Autodesk Inventor part; units mm, degrees
ref_plane "YZ Plane" through (0, 0, 0) normal (1, 0, 0) x (0, 1, 0)
ref_plane "XZ Plane" through (0, 0, 0) normal (0, 1, 0) x (-1, 0, 0)
ref_plane "XY Plane" through (0, 0, 0) normal (0, 0, 1) x (1, 0, 0)
sketch "スケッチ1" plane through (0, 0, 0) normal (0, 0, 1) x (1, 0, 0)
  circle A0 centre (0, 0) radius 1.5
  dimension "d0" = 3
extrude "押し出し1" add sketch "スケッチ1" along normal blind 6
sketch "スケッチ2" plane through (0, 0, 6) normal (0, 0, 1) x (1, 0, 0)
  circle A0 centre (0, 0) radius 1.5
  circle A1 centre (0, 0) radius 3
  dimension "d3" = 6
extrude "押し出し2" add sketch "スケッチ2" along normal blind 2 contours A0 | A1
fillet "フィレット1" radius 2 1 edges at (-3, 0, 8)
thread "ねじ1"
sketch "スケッチ3" plane through (0, 0, 0) normal (0, 0, -1) x (-1, 0, 0)
  circle A0 centre (0, 0) radius 1.5
extrude "押し出し3" add sketch "スケッチ3" along normal blind 9
sketch "スケッチ4" plane through (0, 0, -9) normal (0, 0, -1) x (-1, 0, 0)
  circle A0 centre (0, 0) radius 1.5
extrude "押し出し4" add sketch "スケッチ4" along normal blind 15
properties part number "SB　30mmなべネジ" material "Steel, Mild"
Design review of the part built by this model. Coordinates are the model's own, in mm. A direction names the side the tool comes from. Coordinates: 2 decimals unless noted, no trailing zeros. Loops run counter-clockwise (first coordinate to the right, second up) from the corner with the lowest first, then second, coordinate; pieces in that order, holes last.
Item 1: Add section A-A (z = -2.5). Write out the cut boundary in (x, y), and give its area (3 significant figures).
Completed:
outline: circle Ø3 at (0, 0)
area: 7.07 mm2
Item 2: Clearance check with flat-ended pins moving along their axes: pin 1 (3 mm diameter, centred on x = -1, z = -6.5, fed in from +Y); pin 2 (3 mm diameter, centred on y = -1, z = -3, fed in from -X). State where each tip first meets the part, or that it passes through.
Completed:
pin 1: stops at y = 1.5
pin 2: stops at x = -1.5
Item 3: For faces 1 (the flat face through (0, 0, 8)), 2 (the flat face through (1.3, -1.3, 6)), list the 3-axis set-ups (+Z, -Z, +X, -X, +Y, -Y) from which the entire face can be reached by the end or side of a thin tool; tool diameter is ignored.
Completed:
face 1: +Z, +X, -X, +Y, -Y
face 2: -Z
Item 4: Wall thickness on L1, parallel to Y at x = 0.5, z = -16; L2, parallel to X at y = 1, z = 5; L3, parallel to Z at x = -1, y = 1: over which ranges is each line inside the solid? List them lowest first.
Completed:
L1: y = -1.41 to 1.41
L2: x = -1.12 to 1.12
L3: z = -24 to 7.96
